Part model, mm, in its own coordinate system. Face numbers are marked on the shaded views. Round coordinates to 2 decimals unless told otherwise and drop trailing zeros. Order: outer loops, then holes, each group sorted by start corner. A loop starts at its lowest first (then second) coordinate and runs counter-clockwise, first axis right, second up. Notation, with made-up numbers: (0.25, 89) -> (7.25, 89) arc R28 ccw to (7.25, 116) -> close; hole circle Ø7 at (76, 9). An arc over 180 degrees is marked (long way). Use CSV: the item, a comma, the result in double quotes.
```python
from build123d import *

# Parameters (mm, degrees)
F1_DEPTH = 13
F2_W     = 10
F2_H     = 13
F2_R     = 1.25
F3_DEPTH = 3
F4_DEPTH = 25
F5_R     = 1


with BuildPart() as f1:
    # F0 (on Top) → F1 (new body)
    with BuildSketch(Plane.XY):
        Polygon((-11.62796, 33.897347), (-8.62796, 33.897347), (-8.62796, 39), (-3.52796, 39), (-3.52796, 0), (-0.52796, 0), (-0.52796, 42), (-11.62796, 42), align=None)
    extrude(amount=F1_DEPTH)

    # F2 (on face) → F3 (join)
    with BuildSketch(Plane.YZ.offset(-0.52796)):
        with Locations((5, 6.5)):
            Rectangle(F2_W, F2_H)
        with Locations((5, 6.5)):
            Circle(F2_R, mode=Mode.SUBTRACT)
    extrude(amount=F3_DEPTH)

    # F2 (on face) → F4 (cut)
    with BuildSketch(Plane.YZ.offset(-0.52796)):
        with Locations((5, 6.5)):
            Circle(F2_R)
    extrude(amount=-F4_DEPTH, mode=Mode.SUBTRACT)

    # F5
    f5_edges = [f1.edges().sort_by_distance(p)[0] for p in [
        (-8.62796, 33.897347, 6.5),
        (-3.52796, 0, 6.5),
        (2.47204, 10, 6.5),
        (2.47204, 5, 13),
        (2.47204, 0, 6.5),
        (2.47204, 5, 0),
        (2.47204, 3.75, 6.5),
        (-0.52796, 26, 13),
        (-6.07796, 42, 13),
        (-11.62796, 37.948674, 13),
        (-10.12796, 33.897347, 13),
        (-8.62796, 36.448674, 13),
        (-6.07796, 39, 13),
        (-3.52796, 19.5, 13),
        (-0.52796, 0, 13),
        (0.97204, 10, 13),
        (-6.07796, 42, 0),
        (-11.62796, 37.948674, 0),
        (-10.12796, 33.897347, 0),
        (-8.62796, 36.448674, 0),
        (-6.07796, 39, 0),
        (-3.52796, 19.5, 0),
        (-0.52796, 0, 0),
        (0.97204, 10, 0),
        (-0.52796, 26, 0),
    ]]
    fillet(f5_edges, radius=F5_R)


solid = f1.part
```
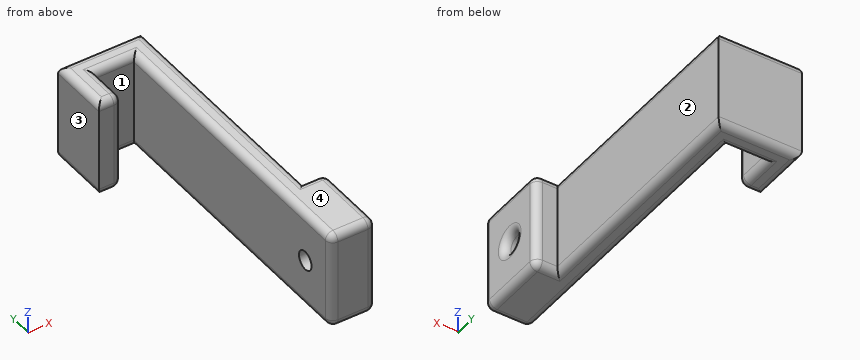
(1) Drop flat-ended pins along their axis: P1, Ø2, axis at y = 4.5, z = 9, coming from the -X side; P2, Ø5.5, axis at y = 31.5, z = 7.5, coming from the +X side; P3, Ø0.6, axis at x = -11, z = 6.5, coming from the -Y side; P4, Ø5, axis at x = -0.5, y = 21.5, coming from the +Z side. Give the stop position or say it passes through.
Reply:
P1,"x = -3.53"
P2,"x = -0.53"
P3,"y = 33.9"
P4,"z = 13"
(2) Cut at B-B, the plane z = 10. Give the cut face in (x, y).
Reply:
outline,"(-11.63, 33.9) -> (-9.63, 33.9) arc R1 ccw to (-8.63, 34.9) -> (-8.63, 39) -> (-3.53, 39) -> (-3.53, 1) arc R1 ccw to (-2.53, 0) -> (1.47, 0) arc R1 ccw to (2.47, 1) -> (2.47, 9) arc R1 ccw to (1.47, 10) -> (-0.53, 10) -> (-0.53, 42) -> (-11.63, 42) -> close"
(3) Probe probe 1 along X at (y, z) = (37.5, 5.25); probe 2 along Z at (x, y) = (-1.2, 5); probe 3 along Y at (x, z) = (-7.75, 3.5). List the from-to ranges inside material, lowest first. Write a range as [from, to].
Reply:
probe 1,"[-11.63, -8.63], [-3.53, -0.53]"
probe 2,"[0, 5.25], [7.75, 13]"
probe 3,"[39, 42]"
(4) Pull direction X, two halves, no side cores. Call the marked faces 1, 2, 3 and 4: released by +X, released by -X, zero draft, split by the parting line, or undercut.
Reply:
face 1,"undercut"
face 2,"released by +X"
face 3,"released by -X"
face 4,"zero draft"
(5) Cut at A-A, the plane y = 5. Give the cut face in (x, z).
Reply:
outline,"(-3.53, 1) arc R1 ccw to (-2.53, 0) -> (1.47, 0) arc R1 ccw to (2.47, 1) -> (2.47, 4.25) arc R1 ccw to (1.47, 5.25) -> (-3.53, 5.25) -> close; (-3.53, 7.75) -> (1.47, 7.75) arc R1 ccw to (2.47, 8.75) -> (2.47, 12) arc R1 ccw to (1.47, 13) -> (-2.53, 13) arc R1 ccw to (-3.53, 12) -> close"
(6) Cut at D-D, the plane x = -8. Give the cut face in (y, z).
Reply:
outline,"(39, 1) arc R1 ccw to (40, 0) -> (41, 0) arc R1 ccw to (42, 1) -> (42, 12) arc R1 ccw to (41, 13) -> (40, 13) arc R1 ccw to (39, 12) -> close"
(7) Cut at C-C, the plane y = 27. Give the cut face in (x, z), then the cut area to 3 significant figures.
Reply:
outline,"(-3.53, 1) arc R1 ccw to (-2.53, 0) -> (-1.53, 0) arc R1 ccw to (-0.53, 1) -> (-0.53, 12) arc R1 ccw to (-1.53, 13) -> (-2.53, 13) arc R1 ccw to (-3.53, 12) -> close"
area,"38.1 mm2"
